CAD build for the part. Positions are in the model's coordinates, mm. A direction names the side the tool comes from. Round coordinates to 2 decimals unless told otherwise and drop trailing zeros. Loops run counter-clockwise (first coordinate to the right, second up) from the corner with the lowest first, then second, coordinate; pieces in that order, holes last. Notation, with made-up numbers: (51.25, -27.75) - (85.25, -27.75) arc R30 ccw to (85.25, 9.25) - close; hole circle Ø3 at (-28.75, 32.25). An arc over 180 degrees is marked (long way). Use one line per item in the form item = value.
from build123d import *

# Parameters (mm, degrees)
BOSS_EXTRUDE1_DEPTH             = 10
BOSS_EXTRUDE2_START             = -3.5
SKETCH2_R                       = 3.5
SKETCH2_R_2                     = 7.5
BOSS_EXTRUDE2_DEPTH             = 3.5
BOSS_EXTRUDE3_REACH             = 247.545
BOSS_EXTRUDE3_DIRECTION_2_DEPTH = 19.65
SKETCH4_R                       = 2.5
CUT_EXTRUDE1_DEPTH              = 248.78291406
SKETCH5_W                       = 120
SKETCH5_H                       = 65
SKETCH5_R                       = 5
BOSS_EXTRUDE4_DEPTH             = 29.65
SKETCH6_W                       = 60
SKETCH6_H                       = 55
CUT_EXTRUDE2_DEPTH              = 19.65


with BuildPart() as part:
    # Sketch1 → Boss-Extrude1 (new body)
    with BuildSketch(Plane(origin=(0, 0, 0), x_dir=(1, 0, 0), z_dir=(0, 1, 0))):
        with BuildLine():
            Line((30, 26.5), (30, -243.5))
            Line((30, -243.5), (-30, -243.5))
            Line((-30, -243.5), (-30, 26.5))
            ThreePointArc((-30, 26.5), (0, 56.5), (30, 26.5))
        make_face()
        with BuildLine():
            ThreePointArc((11.477382224, -17.586065429), (21, 0), (11.477382224, 17.586065429))
            Line((11.477382224, 17.586065429), (5.68518373, 33.5))
            Line((5.68518373, 33.5), (-5.68518373, 33.5))
            Line((-5.68518373, 33.5), (-11.477382224, 17.586065429))
            ThreePointArc((-11.477382224, 17.586065429), (-21, 0), (-11.477382224, -17.586065429))
            Line((-11.477382224, -17.586065429), (-5.68518373, -33.5))
            Line((-5.68518373, -33.5), (5.68518373, -33.5))
            Line((5.68518373, -33.5), (11.477382224, -17.586065429))
        make_face(mode=Mode.SUBTRACT)
    extrude(amount=BOSS_EXTRUDE1_DEPTH)

    # Sketch2 → Boss-Extrude2 (add)
    with BuildSketch(Plane(origin=(0, 10, 0), x_dir=(1, 0, 0), z_dir=(0, 1, 0)).offset(BOSS_EXTRUDE2_START)):
        with BuildLine():
            Line((5.68518373, 33.5), (11.477382224, 17.586065429))
            ThreePointArc((11.477382224, 17.586065429), (21, 0), (11.477382224, -17.586065429))
            Line((11.477382224, -17.586065429), (5.68518373, -33.5))
            Line((5.68518373, -33.5), (-5.68518373, -33.5))
            Line((-5.68518373, -33.5), (-11.477382224, -17.586065429))
            ThreePointArc((-11.477382224, -17.586065429), (-21, 0), (-11.477382224, 17.586065429))
            Line((-11.477382224, 17.586065429), (-5.68518373, 33.5))
            Line((-5.68518373, 33.5), (5.68518373, 33.5))
        make_face()
        with Locations(Location((0, 26.5, 0), (0, 0, 270))):
            Circle(SKETCH2_R, mode=Mode.SUBTRACT)
        with Locations(Location((0, -26.5, 0), (0, 0, 90))):
            Circle(SKETCH2_R, mode=Mode.SUBTRACT)
        with Locations(Location((0, 0, 0), (0, 0, 270))):
            Circle(SKETCH2_R_2, mode=Mode.SUBTRACT)
    extrude(amount=BOSS_EXTRUDE2_DEPTH)

    # Boss-Extrude3: up to this face of the body (flat: up to its plane)
    boss_extrude3_end = Plane(part.part.faces().sort_by_distance((0, 10, 98.054911476))[0])
    # Sketch3 → Boss-Extrude3 (add, up to the picked face)
    with BuildSketch(Plane.XZ, mode=Mode.PRIVATE) as boss_extrude3_sk1:
        with BuildLine():
            Line((35, 243.5), (35, -26.5))
            ThreePointArc((35, -26.5), (0, -61.5), (-35, -26.5))
            Line((-35, -26.5), (-35, 243.5))
            Line((-35, 243.5), (-30, 243.5))
            Line((-30, 243.5), (-30, -26.5))
            ThreePointArc((-30, -26.5), (-29.473014303, -32.09834153), (-27.910571474, -37.5))
            Line((-27.910571474, -37.5), (27.910571474, -37.5))
            ThreePointArc((27.910571474, -37.5), (29.473014303, -32.09834153), (30, -26.5))
            Line((30, -26.5), (30, 243.5))
            Line((30, 243.5), (35, 243.5))
        make_face()
    boss_extrude3_tool1 = split(extrude(boss_extrude3_sk1.sketch, amount=-BOSS_EXTRUDE3_REACH, mode=Mode.PRIVATE), bisect_by=boss_extrude3_end, keep=Keep.BOTH, mode=Mode.PRIVATE)
    add(boss_extrude3_tool1.solids().sort_by(Axis((33.129297, 0, 108.5), (0, 1, 0)))[0])

    # Sketch3 → Boss-Extrude3 direction 2 (add)
    with BuildSketch(Plane.XZ):
        with BuildLine():
            Line((35, 243.5), (35, -26.5))
            ThreePointArc((35, -26.5), (0, -61.5), (-35, -26.5))
            Line((-35, -26.5), (-35, 243.5))
            Line((-35, 243.5), (-30, 243.5))
            Line((-30, 243.5), (-30, -26.5))
            ThreePointArc((-30, -26.5), (-29.473014303, -32.09834153), (-27.910571474, -37.5))
            Line((-27.910571474, -37.5), (27.910571474, -37.5))
            ThreePointArc((27.910571474, -37.5), (29.473014303, -32.09834153), (30, -26.5))
            Line((30, -26.5), (30, 243.5))
            Line((30, 243.5), (35, 243.5))
        make_face()
    extrude(amount=BOSS_EXTRUDE3_DIRECTION_2_DEPTH)

    # Sketch4 → Cut-Extrude1 (cut, through all)
    with BuildSketch(Plane.XZ.offset(19.65)):
        with Locations(Location((-13.955285737, -42.559356041, 0), (0, 0, 270))):
            Circle(SKETCH4_R)
        with Locations(Location((13.955285737, -42.559356041, 0), (0, 0, 270))):
            Circle(SKETCH4_R)
    extrude(amount=-CUT_EXTRUDE1_DEPTH, mode=Mode.SUBTRACT)

    # Sketch5 → Boss-Extrude4 (add)
    with BuildSketch(Plane(origin=(0, 10, 0), x_dir=(1, 0, 0), z_dir=(0, 1, 0))):
        with Locations((0, -274)):
            Rectangle(SKETCH5_W, SKETCH5_H)
        with Locations(Location((46.25, -290.25, 0), (0, 0, 270))):
            Circle(SKETCH5_R, mode=Mode.SUBTRACT)
        with Locations(Location((-46.25, -290.25, 0), (0, 0, 90))):
            Circle(SKETCH5_R, mode=Mode.SUBTRACT)
        with Locations(Location((46.25, -257.75, 0), (0, 0, 90))):
            Circle(SKETCH5_R, mode=Mode.SUBTRACT)
        with Locations(Location((-46.25, -257.75, 0), (0, 0, 270))):
            Circle(SKETCH5_R, mode=Mode.SUBTRACT)
    extrude(amount=-BOSS_EXTRUDE4_DEPTH)

    # Sketch6 → Cut-Extrude2 (cut)
    with BuildSketch(Plane.XZ.offset(19.65)):
        with Locations((0, 269)):
            Rectangle(SKETCH6_W, SKETCH6_H)
    extrude(amount=-CUT_EXTRUDE2_DEPTH, mode=Mode.SUBTRACT)


solid = part.part
1) Slice it at C-C (x = -46.25). Write the cut outline in (y, z), plus the area to 3 significant figures.
Report:
outline = (-19.65, 241.5) - (10, 241.5) - (10, 252.75) - (-19.65, 252.75) - close; (-19.65, 262.75) - (10, 262.75) - (10, 285.25) - (-19.65, 285.25) - close; (-19.65, 295.25) - (10, 295.25) - (10, 306.5) - (-19.65, 306.5) - close
area = 1,330 mm^2
2) Slice it at A-A (x = 0). Write the cut outline in (y, z).
Report:
outline = (-19.65, -61.5) - (10, -61.5) - (10, -30) - (6.5, -30) - (6.5, -33.5) - (0, -33.5) - (0, -37.5) - (-19.65, -37.5) - close; (-19.65, 296.5) - (0, 296.5) - (0, 33.5) - (6.5, 33.5) - (6.5, 30) - (10, 30) - (10, 306.5) - (-19.65, 306.5) - close; (6.5, -23) - (10, -23) - (10, -7.5) - (6.5, -7.5) - close; (6.5, 7.5) - (10, 7.5) - (10, 23) - (6.5, 23) - close
3) Two-plate mould, pull along X, no slides. Class faces 1 (the flat face through (35, -5, 109)), 2 (the flat face through (30, -10, 133)), 3 (the flat face through (-1, 10, 161)): +X half, -X half, draft (parallel to the pull), parting line (faces both ways), or undercut.
Report:
face_1 = +X half
face_2 = undercut
face_3 = draft
4) Flat gauge pins, fed straight in: pin 1 (1.5 mm diameter, centred on y = 6.5, z = 205, fed in from +X); pin 2 (8 mm diameter, centred on x = 4.5, y = 5, fed in from -Z); pin 3 (6 mm diameter, centred on x = -21.5, y = 1, fed in from -Z). Where does each tip first touch, or does it go through?
Report:
pin_1 = 35
pin_2 = -61.5
pin_3 = -56.21
5) Slice it at D-D (y = -10.25). Write the cut outline in (x, z), plus the area to 3 significant figures.
Report:
outline = (-60, 241.5) - (-35, 241.5) - (-35, -26.5) arc R35 ccw to (35, -26.5) - (35, 241.5) - (60, 241.5) - (60, 306.5) - (-60, 306.5) - close; hole circle Ø10 at (-46.25, 257.75); hole circle Ø10 at (-46.25, 290.25); hole (-30, -26.5) arc R30 ccw to (-27.91, -37.5) - (27.91, -37.5) arc R30 ccw to (30, -26.5) - (30, 296.5) - (-30, 296.5) - close; hole circle Ø5 at (-13.96, -42.56); hole circle Ø5 at (13.96, -42.56); hole circle Ø10 at (46.25, 257.75); hole circle Ø10 at (46.25, 290.25)
area = 8,110 mm^2
6) Drill centre lines: probe 1 along X at (y, z) = (-5.25, 290.25); probe 2 along X at (y, z) = (-0.5, 141.5); probe 3 along Z at (x, y) = (42, -7.5). Where is each one in solid material? Low to high.
Report:
probe_1 = -60 to -51.25, -41.25 to -30, 30 to 41.25, 51.25 to 60
probe_2 = -35 to -30, 30 to 35
probe_3 = 241.5 to 255.12, 260.38 to 287.62, 292.88 to 306.5
7) Tool access for faces 4 (the flat face through (-35, -5, 106)), 5 (the flat face through (0, 3, -33.5)), 6 (the flat face through (47, -5, 241.5)), 7 (the cylindrical face through (47.75, -4.62, 295.02)): list every direction of +Z, -Z, +X, -X, +Y, -Y with a clear straight run to the whole face (end or side of a thin tool).
Report:
face_4 = -Z, -X, +Y, -Y
face_5 = -Y
face_6 = -Z, +X, +Y, -Y
face_7 = +Y, -Y
8) Slice it at B-B (z = 191). Write the cut outline in (x, y).
Report:
outline = (-35, -19.65) - (-30, -19.65) - (-30, 0) - (30, 0) - (30, -19.65) - (35, -19.65) - (35, 10) - (-35, 10) - close
